from build123d import *

# Parameters (mm, degrees)
ESBO_O1_R                = 8
RESSALTO_EXTRUS_O1_DEPTH = 13
CORTE_EXTRUS_O1_START    = -10
CORTE_EXTRUS_O1_DEPTH    = 10
PADR_OCIRCULAR1_COUNT    = 10
ESBO_O5_R                = 2.75
CORTE_EXTRUS_O2_DEPTH    = 2.5
FILETE1_R                = 1


with BuildPart() as part:
    # Esboço1 → Ressalto-extrusão1 (new body)
    with BuildSketch(Plane.XY.offset(-62.474592215)):
        with Locations(Location((154.344666384, -4.979841337, 0), (0, 0, 90))):
            Circle(ESBO_O1_R)
        with BuildLine():
            Line((156.839244486, -3.946845648), (152.817363907, -2.753331256))
            ThreePointArc((152.817363907, -2.753331256), (151.756235333, -4.211710693), (151.850088282, -6.012837026))
            Line((151.850088282, -6.012837026), (155.871968862, -7.206351418))
            ThreePointArc((155.871968862, -7.206351418), (156.933097439, -5.747971979), (156.839244486, -3.946845648))
        make_face(mode=Mode.SUBTRACT)
    extrude(amount=RESSALTO_EXTRUS_O1_DEPTH)

    # Esboço4 → Corte-extrusão1 (cut)
    with BuildSketch(Plane.XY.offset(-49.474592215).offset(CORTE_EXTRUS_O1_START)):
        with BuildLine():
            Line((155.259844023, -10.698578623), (155.334666384, -11.166126571))
            ThreePointArc((155.334666384, -11.166126571), (155.355864946, -11.365142474), (155.389666384, -11.562409225))
            ThreePointArc((155.389666384, -11.562409225), (155.798933371, -12.200119109), (156.344666384, -12.725808029))
            ThreePointArc((156.344666384, -12.725808029), (154.344666384, -12.979841337), (152.344666384, -12.725808029))
            ThreePointArc((152.344666384, -12.725808029), (152.890399398, -12.200119109), (153.299666384, -11.562409225))
            ThreePointArc((153.299666384, -11.562409225), (153.333467823, -11.365142474), (153.354666384, -11.166126571))
            Line((153.354666384, -11.166126571), (153.470297344, -10.443574954))
            ThreePointArc((153.470297344, -10.443574954), (153.591194582, -10.240482514), (153.8185158, -10.175769725))
            ThreePointArc((153.8185158, -10.175769725), (154.225958814, -10.20099205), (154.634127125, -10.194313384))
            ThreePointArc((154.634127125, -10.194313384), (155.043877847, -10.326217347), (155.259844023, -10.698578623))
        make_face()
    corte_extrus_o1 = extrude(amount=CORTE_EXTRUS_O1_DEPTH, mode=Mode.SUBTRACT)

    # PadrãoCircular1: Corte-extrusão1 ×10 about axis
    padr_ocircular1_axis = Axis((154.344666384, -4.979841337, 0), (0, 0, 1))
    for i in range(1, PADR_OCIRCULAR1_COUNT):
        add(corte_extrus_o1.rotate(padr_ocircular1_axis, i * 360 / PADR_OCIRCULAR1_COUNT), mode=Mode.SUBTRACT)

    # Esboço5 → Corte-extrusão2 (cut)
    with BuildSketch(Plane(origin=(0, 0, -62.474592215), x_dir=(-1, 0, 0), z_dir=(0, 0, -1))):
        with Locations((-154.344666384, -4.979841337)):
            Circle(ESBO_O5_R)
    extrude(amount=-CORTE_EXTRUS_O2_DEPTH, mode=Mode.SUBTRACT)

    # Filete1
    # the kernel refuses this fillet: 1 mm, written as the material it adds along each edge
    with BuildSketch(Plane(origin=(154.344666384, -4.979841337, -59.974592215), x_dir=(-1, 0, 0), z_dir=(0, -1, 0))) as filete1_piece_1_section:
        with BuildLine():
            CenterArc((2.75 - FILETE1_R, FILETE1_R), FILETE1_R, 270, 90)
            Line((2.75 - FILETE1_R, 0), (2.75, 0))
            Line((2.75, 0), (2.75, FILETE1_R))
        make_face()
    filete1_piece_1 = revolve(axis=Axis((154.344666384, -4.979841337, -59.974592215), (0, 0, -1)), mode=Mode.PRIVATE)
    filete1_piece_1 = filete1_piece_1 - Plane(origin=(154.344666389, -4.979841339, -60.815647373), x_dir=(-0.5656675853449286, 0.8246333627073538, 0), z_dir=(0, 0, -1)) * Cylinder(2.700000004, 12, mode=Mode.PRIVATE)
    add(filete1_piece_1)
    with BuildSketch(Plane(origin=(154.344666384, -4.979841337, -59.974592215), x_dir=(-1, 0, 0), z_dir=(0, -1, 0))) as filete1_piece_2_section:
        with BuildLine():
            CenterArc((2.75 - FILETE1_R, FILETE1_R), FILETE1_R, 270, 90)
            Line((2.75 - FILETE1_R, 0), (2.75, 0))
            Line((2.75, 0), (2.75, FILETE1_R))
        make_face()
    filete1_piece_2 = revolve(axis=Axis((154.344666384, -4.979841337, -59.974592215), (0, 0, -1)), mode=Mode.PRIVATE)
    filete1_piece_2 = split(filete1_piece_2, bisect_by=Plane(origin=(154.828304199, -3.350088453, -60.157362132), z_dir=(0.28449283065041153, 0.9586781677437514, 0)), keep=Keep.TOP, mode=Mode.PRIVATE)
    add(filete1_piece_2)
    with BuildSketch(Plane(origin=(154.344666384, -4.979841337, -59.974592215), x_dir=(-1, 0, 0), z_dir=(0, -1, 0))) as filete1_piece_3_section:
        with BuildLine():
            CenterArc((2.75 - FILETE1_R, FILETE1_R), FILETE1_R, 270, 90)
            Line((2.75 - FILETE1_R, 0), (2.75, 0))
            Line((2.75, 0), (2.75, FILETE1_R))
        make_face()
    filete1_piece_3 = revolve(axis=Axis((154.344666384, -4.979841337, -59.974592215), (0, 0, -1)), mode=Mode.PRIVATE)
    filete1_piece_3 = split(filete1_piece_3, bisect_by=Plane(origin=(152.118883506, -6.092603434, -60.089217232), z_dir=(-0.284492830650411, -0.9586781677437516, 0)), keep=Keep.TOP, mode=Mode.PRIVATE)
    add(filete1_piece_3)


solid = part.part
Geometry: final body of the model. Coordinates: model frame, mm. A direction names the side the tool comes from. Give positions to 0.01 mm unless a question says otherwise; leave off trailing zeros. Loops run counter-clockwise (first coordinate to the right, second up) from the corner with the lowest first, then second, coordinate; pieces in that order, holes last. Notation, with made-up numbers: M -25.5,7 L -3.5,7 A36 ccw -3.5,44 Z; hole C -1.75,-36.75 d2. An arc over 180 degrees is marked long. Put each result on its own line as item: value. Start each with the question number.
1) Pull-direction query (Y, two-part tool) for faces 1 (the flat face through (158, -5, -62.475)), 2 (the cylindrical face through (152.88, -12.21, -54.54)), 3 (the cylindrical face through (147.921, -1.357, -54.545)), 4 (the cylindrical face through (152.9, 2.23, -54.54)); classes: pulls with the +Y half, pulls with the -Y half, needs draft (parallel to the pull), parting line crosses it, or undercut.
2) Access query for faces 5 (the cylindrical face through (151.722, -4.154, -61.735)), 6 (the cylindrical face through (151.277, -11.665, -54.545)), 7 (the cylindrical face through (159.78, 0.01, -54.54)), 8 (the cylindrical face through (160.768, -8.603, -54.545)). Directions: +Z, -Z, +X, -X, +Y, -Y. A direction counts if a zero-diameter tool reaches every point of the face in a straight line with its end or side. Return the directions, or none.
3) Ray query, line 1 along Y through (x, z) = (159.5, -54); line 2 along Y through (x, z) = (160, -52.75); line 3 along X through (y, z) = (-11, -51.5). Return the intervals inside material, ascending.
4) Cut plane A-A (z = -61.5). Output: boundary loops of the cut face in (x, y).
5) Contact query for flat-ended pins moving along their axis: pin 1 (1.1 mm diameter, centred on x = 150.5, y = -10.5, fed in from +Z); pin 2 (1 mm diameter, centred on y = -7, z = -59.5, fed in from -X); pin 3 (3 mm diameter, centred on y = -10.5, z = -54, fed in from +X). Output: stop coordinate, or through.
Verdict:
1. face 1: needs draft
1. face 2: pulls with the -Y half
1. face 3: undercut
1. face 4: pulls with the +Y half
2. face 5: -Z
2. face 6: +Z, -X
2. face 7: +Z, +Y
2. face 8: +Z, +X
3. line 1: -9.88 to -7.62, -6.1 to -3.99, -2.34 to -0.07
3. line 2: -10.02 to -7.87, -5.87 to -4.09, -2.09 to 0.06
3. line 3: 151.31 to 153.38, 155.31 to 157.38
4. outline: C 154.34,-4.98 d16; hole C 154.34,-4.98 d5.5
5. pin 1: z = -59.47
5. pin 2: x = 146.49
5. pin 3: x = 161.09
